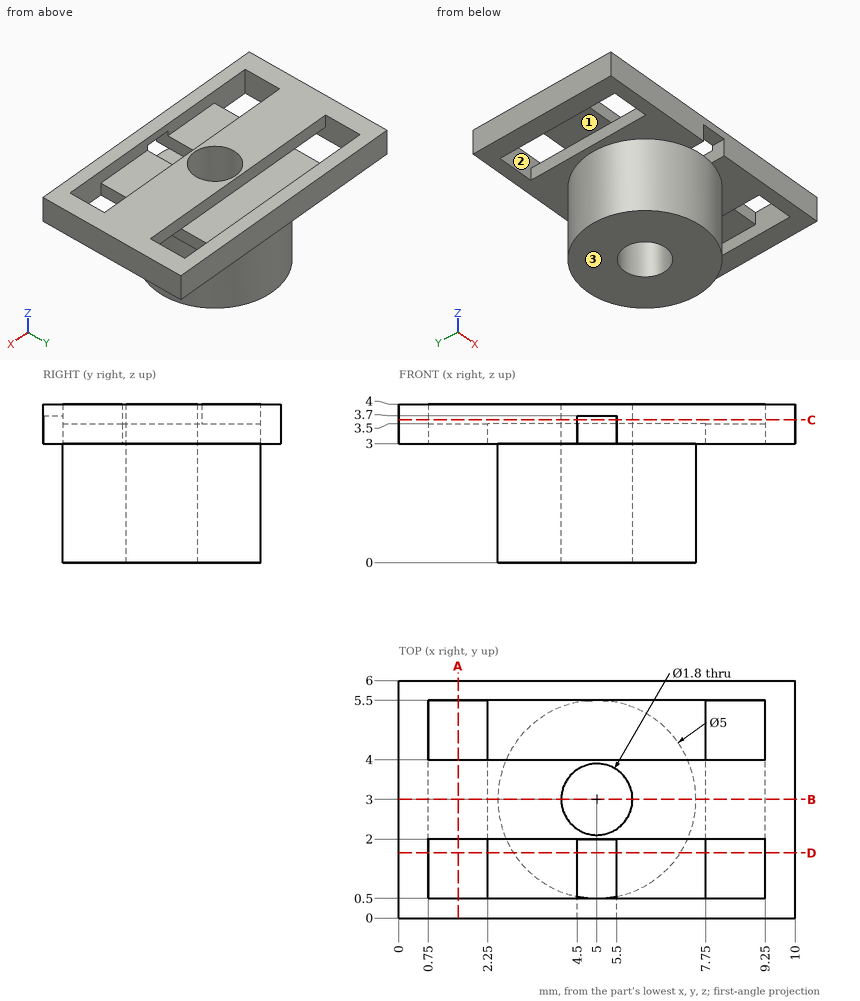
Here's the drawing with two shaded views (mm, measured from the low corner). I have some questions. A direction names the side the tool comes from. Coordinates: 2 decimals unless noted, no trailing zeros. Order: outer loops, then holes, each group sorted by start corner. A loop starts at its lowest first (then second) coordinate and runs counter-clockwise, first axis right, second up. Notation, with made-up numbers: (81.25, 49) - (132.25, 49) arc R20 cw to (132.25, 65) - close; hole circle Ø8 at (33.5, -24). An arc over 180 degrees is marked (long way). Answer in a Markdown table with one row per item. Add a question column.
(1) If we section it at D-D, the plane y = 1.65: Please give me the cut outline in (x, z), then the cut area to 3 significant figures.
(2) If we section it at C-C, the plane z = 3.6: Please give me the cut outline in (x, y), then the cut area to 3 significant figures.
(3) I need wall thicknesses on L1, parallel to Y at x = 5, z = 2.35; L2, parallel to Z at x = 2.5, y = 1.55; L3, parallel to Z at x = 9.5, y = 5.4. Which ranges of each line are inside material? Lowest first, please.
(4) Will this pin go through, and if not, where does the flat tip stop? pin 1 (1.6 mm diameter, centred on x = 1, y = 3, fed in from -Z).
(5) If we section it at A-A, the plane x = 1.5: Please give me the cut outline in (y, z), then the cut area to 3 significant figures.
(6) On a 3-axis mill with a long thin cutter (end or side, diameter ignored), from which of +Z, -Z, +X, -X, +Y, -Y can I reach the whole of each face in a straight line? I mean the marked faces 1, 2 and 3. Say none if no direction works.
(7) If we section it at B-B, the plane y = 3: Please give me the cut outline in (x, z).
Results are:
| question | item | result |
|---|---|---|
| 1 | outline | (0, 3) - (0.75, 3) - (0.75, 4) - (0, 4) - close; (2.25, 3) - (2.9, 3) - (2.9, 0) - (7.1, 0) - (7.1, 3) - (7.75, 3) - (7.75, 3.5) - (5.5, 3.5) - (5.5, 3) - (4.5, 3) - (4.5, 3.5) - (2.25, 3.5) - close; (9.25, 3) - (10, 3) - (10, 4) - (9.25, 4) - close |
| 1 | area | 16.4 mm2 |
| 2 | outline | (0, 0) - (4.5, 0) - (4.5, 0.5) - (0.75, 0.5) - (0.75, 2) - (9.25, 2) - (9.25, 0.5) - (5.5, 0.5) - (5.5, 0) - (10, 0) - (10, 6) - (0, 6) - close; hole (0.75, 4) - (9.25, 4) - (9.25, 5.5) - (0.75, 5.5) - close; hole circle Ø1.8 at (5, 3) |
| 2 | area | 31.5 mm2 |
| 3 | L1 | y = 0.5 to 2.1, 3.9 to 5.5 |
| 3 | L2 | z = 3 to 3.5 |
| 3 | L3 | z = 3 to 4 |
| 4 | pin 1 | stops at z = 3 |
| 5 | outline | (0, 3) - (0.5, 3) - (0.5, 4) - (0, 4) - close; (2, 3.5) - (4, 3.5) - (4, 4) - (2, 4) - close; (5.5, 3) - (6, 3) - (6, 4) - (5.5, 4) - close |
| 5 | area | 2.00 mm2 |
| 6 | face 1 | -Z |
| 6 | face 2 | +Z |
| 6 | face 3 | -Z, +X, -X, +Y, -Y |
| 7 | outline | (0, 3) - (0.75, 3) - (0.75, 3.5) - (2.25, 3.5) - (2.25, 3) - (2.5, 3) - (2.5, 0) - (4.1, 0) - (4.1, 4) - (0, 4) - close; (5.9, 0) - (7.5, 0) - (7.5, 3) - (7.75, 3) - (7.75, 3.5) - (9.25, 3.5) - (9.25, 3) - (10, 3) - (10, 4) - (5.9, 4) - close |
